Geometry: see drawing. Coordinates: mm, zero at the bounding-box minimum. A direction names the side the tool comes from. Coordinates: 2 decimals unless noted, no trailing zeros. Order: outer loops, then holes, each group sorted by start corner. A loop starts at its lowest first (then second) coordinate and runs counter-clockwise, first axis right, second up. Notation, with made-up numbers: M 21,50 L 52,50 A21 cw 52,54 Z; hole C -39.75,-19 d1. An arc over 180 degrees is marked long. Answer in a Markdown table with one row per item.
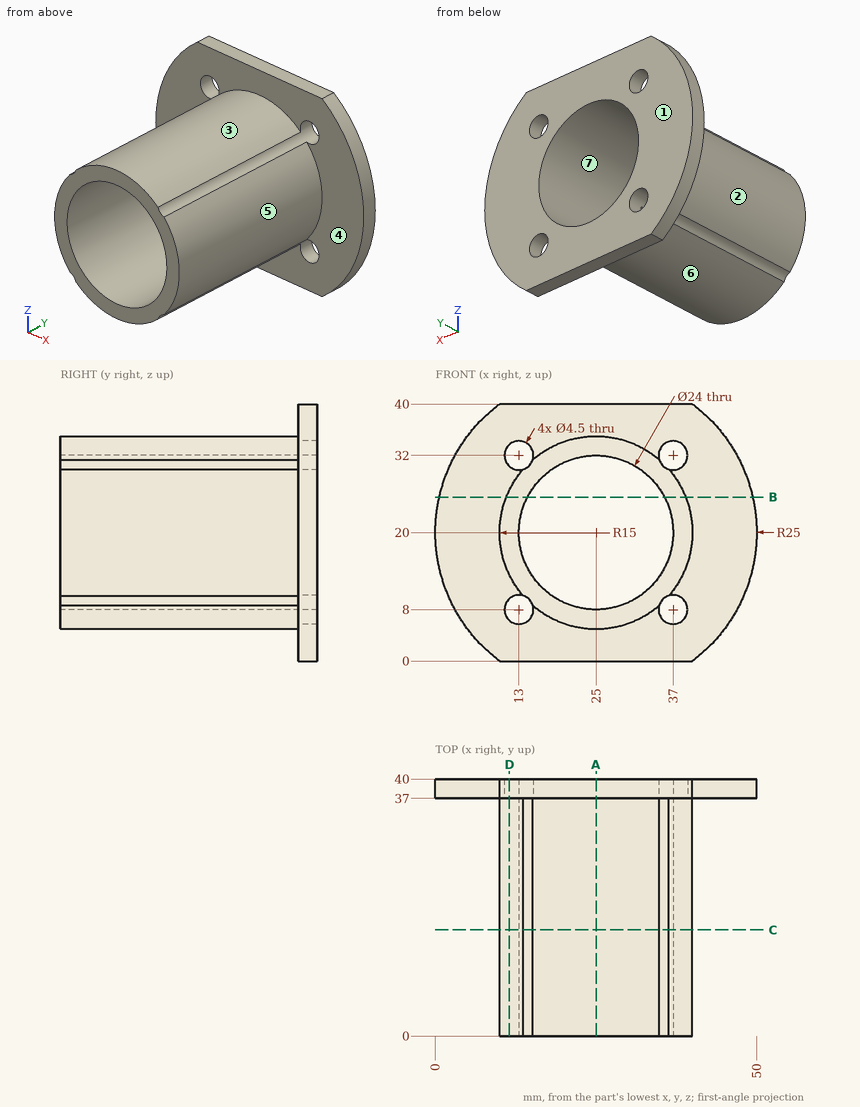
1) Cut plane D-D, the plane x = 11.5. Output: boundary loops of the cut face in (y, z).
Resolved:
| item | result |
|---|---|
| outline | M 0,13.46 L 37,13.46 L 37,9.68 L 40,9.68 L 40,30.32 L 37,30.32 L 37,26.54 L 0,26.54 Z; M 37,0 L 40,0 L 40,6.32 L 37,6.32 Z; M 37,33.68 L 40,33.68 L 40,40 L 37,40 Z |
2) Material intervals for probe 1 along Y at (x, z) = (44, 36); probe 2 along X at (y, z) = (22, 23); probe 3 along X at (y, z) = (13, 13), sorted ascending.
Resolved:
| item | result |
|---|---|
| probe 1 | y = 37 to 40 |
| probe 2 | x = 10.3 to 13.38, 36.62 to 39.7 |
| probe 3 | x = 11.73 to 15.25, 34.75 to 38.27 |
3) Cut plane C-C, the plane y = 16.5. Output: boundary loops of the cut face in (x, z), and give its area (3 significant figures).
Resolved:
| item | result |
|---|---|
| outline | M 13.7,10.14 A2.25 cw 15.14,8.7 A15 ccw 34.86,8.7 A2.25 cw 36.3,10.14 A15 ccw 36.3,29.86 A2.25 cw 34.86,31.3 A15 ccw 15.14,31.3 A2.25 cw 13.7,29.86 A15 ccw Z; hole C 25,20 d24 |
| area | 253 mm2 |
4) Mould query, pull axis Z, two halves, no side actions, for the marked faces 4, 5, 6 and 7. Classes: +Z half, -Z half, draft (parallel to the pull), parting line (faces both ways), or undercut.
Resolved:
| item | result |
|---|---|
| face 4 | draft |
| face 5 | parting line |
| face 6 | -Z half |
| face 7 | undercut |
5) Reachability of the marked faces 1, 2 and 3 from +Z, -Z, +X, -X, +Y, -Y: full face, straight path, thin tool, end or side. Return the list, or none.
Resolved:
| item | result |
|---|---|
| face 1 | +Z, -Z, +X, -X, +Y |
| face 2 | -X, -Y |
| face 3 | +Z, -Y |
6) Cut plane A-A, the plane x = 25. Output: boundary loops of the cut face in (y, z), and give its area (3 significant figures).
Resolved:
| item | result |
|---|---|
| outline | M 0,5 L 37,5 L 37,0 L 40,0 L 40,8 L 0,8 Z; M 0,32 L 40,32 L 40,40 L 37,40 L 37,35 L 0,35 Z |
| area | 270 mm2 |
7) Contact query for flat-ended pins moving along their axis: pin 1 (12 mm diameter, centred on x = 34, z = 28, fed in from -Y); pin 2 (4 mm diameter, centred on x = 37.5, y = 4, fed in from -Z); pin 3 (1 mm diameter, centred on x = 30, y = 35.5, fed in from -Z); pin 4 (1 mm diameter, centred on y = 32, z = 8, fed in from -X). Output: stop coordinate, or through.
Resolved:
| item | result |
|---|---|
| pin 1 | stops at y = 0 |
| pin 2 | stops at z = 9.68 |
| pin 3 | stops at z = 5.69 |
| pin 4 | stops at x = 15.37 |
8) Cut plane B-B, the plane z = 25.5. Output: boundary loops of the cut face in (x, y).
Resolved:
| item | result |
|---|---|
| outline | M 0.61,37 L 11.04,37 L 11.04,0 L 14.33,0 L 14.33,40 L 0.61,40 Z; M 35.67,0 L 38.96,0 L 38.96,37 L 49.39,37 L 49.39,40 L 35.67,40 Z |
